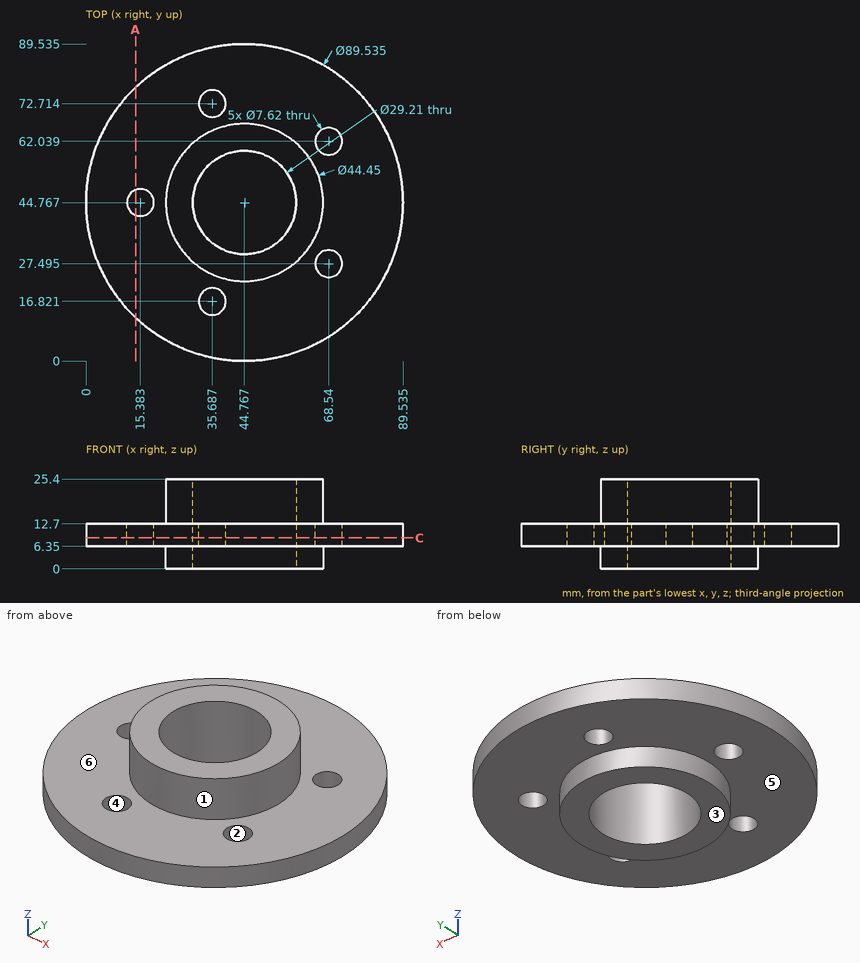
Answer from the drawing. Dimensions are ordinates in mm from the lowest x, y and z of the part. A direction names the side the tool comes from. Coordinates: 2 decimals unless noted, no trailing zeros. Write each loop counter-clockwise with the first axis right and the second up, starting at its lowest first coordinate (ties: lowest second). Pieces come first, ordered by that corner, then holes. Notation, with made-up numbers: (9.5, 7.5) - (42.5, 7.5) arc R18 cw to (42.5, 36.5) - close; hole circle Ø10 at (79, -10). An arc over 180 degrees is marked (long way). Answer as CSV lines item,"result".
1. Find section A-A (x = 14). Give the vertices of the cut face in (y, z).
Computed values:
outline,"(12.25, 6.35) - (41.22, 6.35) - (41.22, 12.7) - (12.25, 12.7) - close; (48.32, 6.35) - (77.29, 6.35) - (77.29, 12.7) - (48.32, 12.7) - close"
2. Determine the mould class of the marked faces 1, 2 and 3 for opening direction Y: +Y half, -Y half, draft (parallel to the pull), parting line (faces both ways), or undercut.
Computed values:
face 1,"parting line"
face 2,"undercut"
face 3,"draft"
3. Find section C-C (z = 8.75). Give the number of separate pieces and of enclosed holes in the cut face, plus the area to 3 significant figures.
Computed values:
separate pieces,"1"
enclosed holes,"6"
area,"5,400 mm²"
4. Straight lines are drawn through the part: line 1 (Z direction, x = 74, y = 47.5); line 2 (Y direction, x = 44, z = 6) (1 decimal); line 3 (X direction, y = 34, z = 12) (1 decimal). For each, find the intervals that lie inside material, in ascending order. Write a range as [from, to].
Computed values:
line 1,"z = [6.35, 12.7]"
line 2,"y = [22.6, 30.2], [59.4, 67]"
line 3,"x = [1.3, 34.9], [54.6, 88.2]"
5. Given P1, Ø12, axis at x = 35.69, y = 72.71, coming from the -Z side; P2, Ø6, axis at x = 35.69, y = 16.82, coming from the -Z side; P3, Ø2, axis at x = 49, y = 76, coming from the +Z side; P4, Ø1.5, axis at x = 27, z = 8.5, coming from the -Y side, each flat-ended and moving along its own axis, determine where each tip first touches the part or whether it passes through.
Computed values:
P1,"stops at z = 6.35"
P2,"passes through"
P3,"stops at z = 12.7"
P4,"stops at y = 3.36"
6. A tool of negligible diameter and unlimited length cuts with its end or side. For the marked faces 4, 5 and 6, from which of +Z, -Z, +X, -X, +Y, -Y can it reach the whole face along a straight path? Write none if from no direction.
Computed values:
face 4,"+Z, -Z"
face 5,"-Z"
face 6,"+Z"
